Verification items for the finished model (mm, model axes). A direction names the side the tool comes from. Coordinates: 2 decimals unless noted, no trailing zeros. Order: outer loops, then holes, each group sorted by start corner. A loop starts at its lowest first (then second) coordinate and runs counter-clockwise, first axis right, second up. Notation, with made-up numbers: (44.5, 44) -> (54.5, 44) arc R34 ccw to (54.5, 76) -> close; hole circle Ø7 at (10.5, -13). An arc over 180 degrees is marked (long way). Write each question's results on one line, items separated by ' | '. Start each with the question number.
(1) Set-up check for faces 1 (the cylindrical face through (7.136, -3.79, 20.767)), 2 (the flat face through (-2, -12, -19.45)), 3 (the flat face through (8, -12, -17.45)): record each of +Z, -Z, +X, -X, +Y, -Y from which the full face is reachable in a straight line by a thin tool's end or side.
(2) Thickness scan on probe 1 along Y at (x, z) = (7.91, 20.9); probe 2 along Y at (x, z) = (4.75, -4.5); probe 3 along Z at (x, y) = (-3.25, -12). Record the ranges inside material, lowest first. Write a range as [from, to].
(3) Cross-section at B-B on x = 7.91. Enter the section's corners in (y, z).
(4) Cross-section at A-A on y = -20.4. Enter the section's corners in (x, z).
(5) Cross-section at D-D on y = -12.45. Enter the section's corners in (x, z).
(6) Draft check along X on faces 4 (the cylindrical face through (7.08, -21.04, 20.77)), 5 (the flat face through (5, -12, 21.95)), 6 (the cylindrical face through (7.16, -12.55, -18.44)), 7 (the cylindrical face through (-0.767, -13.457, -27.485)). Enter one of: +X half, -X half, draft (parallel to the pull), parting line (faces both ways), or undercut.
(7) Go/stop test with flat-tipped pins: pin 1 (1 mm diameter, centred on y = -3.5, z = -18, fed in from -X); pin 2 (2.5 mm diameter, centred on x = 7.91, y = -4.5, fed in from -Z); pin 3 (5.5 mm diameter, centred on x = 6, y = -11, fed in from -Z); pin 4 (10 mm diameter, centred on y = -13.5, z = 11.5, fed in from +X). Record where each tip stops, or that it passes through.
(8) Cross-section at C-C on z = -4.5. Enter the section's corners in (x, y), and give its area (3 significant figures).
```python
from build123d import *

# Parameters (mm, degrees)
F1_DEPTH  = 24.9
F2_W      = 19.9
F2_H      = 36.5
F3_DEPTH  = 25.4
F4_W      = 24.9
F4_H      = 5
F4_H_2    = 7.5
F5_DEPTH  = 2.5
F7_DEPTH  = 2.5
F8_R      = 1.05
F9_DEPTH  = 25.4
F10_R     = 4.699
F11_DEPTH = 8
F12_R     = 1.016
F13_DEPTH = 5
F14_W     = 2.5
F14_H     = 7.5
F14_H_2   = 5
F15_DEPTH = 25.4
F17_DEPTH = 25.4
F18_W     = 5.8
F18_H     = 19.9
F19_DEPTH = 0.5


with BuildPart() as f1:
    # F0 (on Front) → F1 (new body)
    with BuildSketch(Plane.XZ):
        Polygon((10.16, 21.95), (0, 21.95), (-10.16, 21.95), (-10.16, -21.95), (10.16, -21.95), (10.16, 0), align=None)
    extrude(amount=F1_DEPTH)

    # F2 (on face) → F3 (cut)
    with BuildSketch(Plane(origin=(-10.16, 0, 0), x_dir=(0, -1, 0), z_dir=(-1, 0, 0))):
        with Locations((12.45, 1.3)):
            Rectangle(F2_W, F2_H)
    extrude(amount=-F3_DEPTH, mode=Mode.SUBTRACT)

    # F4 (on face) → F5 (join)
    with BuildSketch(Plane(origin=(-10.16, 0, 0), x_dir=(0, -1, 0), z_dir=(-1, 0, 0))):
        with Locations((12.45, 19.45)):
            Rectangle(F4_W, F4_H)
        with Locations((12.45, -18.2)):
            Rectangle(F4_W, F4_H_2)
    extrude(amount=F5_DEPTH)

    # F6 (on face) → F7 (cut)
    with BuildSketch(Plane.XY.offset(-16.95)):
        with BuildLine():
            Line((4.36, -6.370526), (4.36, -2.5))
            Line((4.36, -2.5), (-10.16, -2.5))
            Line((-10.16, -2.5), (-10.16, -22.4))
            Line((-10.16, -22.4), (4.36, -22.4))
            Line((4.36, -22.4), (4.36, -18.529474))
            ThreePointArc((4.36, -18.529474), (7.16, -12.45), (4.36, -6.370526))
        make_face()
    extrude(amount=-F7_DEPTH, mode=Mode.SUBTRACT)

    # F8 (on face) → F9 (cut)
    with BuildSketch(Plane.XY.offset(21.95)):
        with Locations((7.91, -4.5)):
            Circle(F8_R)
        with Locations((7.91, -20.4)):
            Circle(F8_R)
    extrude(amount=-F9_DEPTH, mode=Mode.SUBTRACT)

    # F10 (on face) → F11 (join)
    with BuildSketch(Plane(origin=(0, 0, -21.95), x_dir=(1, 0, 0), z_dir=(0, 0, -1))):
        with Locations((-0.635, 12.45)):
            Circle(F10_R)
    extrude(amount=F11_DEPTH)

    # F12 (on face) → F13 (cut)
    with BuildSketch(Plane(origin=(0, 0, -29.95), x_dir=(1, 0, 0), z_dir=(0, 0, -1))):
        with Locations((-0.635, 12.45)):
            Circle(F12_R)
    extrude(amount=-F13_DEPTH, mode=Mode.SUBTRACT)

    # F14 (on face) → F15 (cut)
    with BuildSketch(Plane.XZ.offset(24.9)):
        with Locations((-11.41, -18.2)):
            Rectangle(F14_W, F14_H)
        with Locations((-11.41, 19.45)):
            Rectangle(F14_W, F14_H_2)
    extrude(amount=-F15_DEPTH, mode=Mode.SUBTRACT)

    # F16 (on face) → F17 (cut)
    with BuildSketch(Plane(origin=(0, 0, 0), x_dir=(-1, 0, 0), z_dir=(0, 1, 0))):
        Polygon((10.16, 21.95), (0, 21.95), (10.16, 0), align=None)
    extrude(amount=-F17_DEPTH, mode=Mode.SUBTRACT)

    # F18 (on face) → F19 (cut)
    with BuildSketch(Plane.XY.offset(-16.95)):
        with Locations((7.26, -12.45)):
            Rectangle(F18_W, F18_H)
    extrude(amount=-F19_DEPTH, mode=Mode.SUBTRACT)


solid = f1.part
```
Results are:
1) face 1: +Z | face 2: -X | face 3: +X, -X
2) probe 1: y = [-24.9, -21.45], [-19.35, -5.55], [-3.45, 0] | probe 2: y = [-24.9, -22.4], [-2.5, 0] | probe 3: z = [-29.95, -19.45]
3) outline: (-24.9, -21.95) -> (0, -21.95) -> (0, 21.95) -> (-3.45, 21.95) -> (-3.45, 19.55) -> (-2.5, 19.55) -> (-2.5, -17.45) -> (-22.4, -17.45) -> (-22.4, 19.55) -> (-21.45, 19.55) -> (-21.45, 21.95) -> (-24.9, 21.95) -> close; (-19.35, 19.55) -> (-5.55, 19.55) -> (-5.55, 21.95) -> (-19.35, 21.95) -> close
4) outline: (-10.16, -21.95) -> (10.16, -21.95) -> (10.16, -17.45) -> (4.36, -17.45) -> (4.36, -19.45) -> (-10.16, -19.45) -> close; (-1.11, 19.55) -> (6.86, 19.55) -> (6.86, 21.95) -> (0, 21.95) -> close; (8.96, 19.55) -> (10.16, 19.55) -> (10.16, 21.95) -> (8.96, 21.95) -> close
5) outline: (-10.16, -21.95) -> (-5.33, -21.95) -> (-5.33, -29.95) -> (-1.65, -29.95) -> (-1.65, -24.95) -> (0.38, -24.95) -> (0.38, -29.95) -> (4.06, -29.95) -> (4.06, -21.95) -> (10.16, -21.95) -> (10.16, -17.45) -> (7.16, -17.45) -> (7.16, -19.45) -> (-10.16, -19.45) -> close; (-1.11, 19.55) -> (10.16, 19.55) -> (10.16, 21.95) -> (0, 21.95) -> close
6) face 4: undercut | face 5: draft | face 6: -X half | face 7: undercut
7) pin 1: stops at x = 4.36 | pin 2: stops at z = -21.95 | pin 3: stops at z = -29.95 | pin 4: passes through
8) outline: (-10.16, -24.9) -> (10.16, -24.9) -> (10.16, -22.4) -> (-10.16, -22.4) -> close; (-10.16, -2.5) -> (10.16, -2.5) -> (10.16, 0) -> (-10.16, 0) -> close | area: 102 mm2
